Source: CAD feature listing. Evaluate the final solid. Frame: model axes, mm. A direction names the side the tool comes from. Round coordinates to 2 decimals unless told otherwise and drop trailing zeros. Loops run counter-clockwise (first coordinate to the right, second up) from the corner with the lowest first, then second, coordinate; pieces in that order, holes last. Notation, with made-up numbers: (84, 40) -> (89, 40) arc R12 ccw to (89, 61) -> close; hole circle Ø1 at (15.5, 87.5). An arc over 180 degrees is marked (long way). Write item = value, one per line.
from build123d import *

# Parameters (mm, degrees)
F0_W     = 41.6900217533
F0_H     = 40.332518518
F1_DEPTH = 560
F2_DEPTH = 600
F3_DEPTH = 2000
F4_T     = -18


with BuildPart() as f1:
    # F0 (on Front) → F1 (new body)
    with BuildSketch(Plane.XZ):
        with Locations((20.8450108767, 20.166259259)):
            Rectangle(F0_W, F0_H)
    extrude(amount=F1_DEPTH)

    # F2 (add): a face of the model
    f2_faces = [f1.faces().sort_by_distance(p)[0] for p in [
        (0, -280, 20.166259259),
    ]]
    extrude(f2_faces, amount=-F2_DEPTH)

    # F3 (add): a face of the model
    f3_faces = [f1.faces().sort_by_distance(p)[0] for p in [
        (300, -280, 0),
    ]]
    extrude(f3_faces, amount=-F3_DEPTH)

    # F4
    f4_openings = [f1.faces().sort_by_distance(p)[0] for p in [
        (300, -560, 1000),
    ]]
    offset(amount=F4_T, openings=f4_openings)


solid = f1.part
1. Section query A-A (z = 1758.5). Return the cut outline in (x, y), then the cut area to 3 significant figures.
Evaluation:
outline = (0, -560) -> (18, -560) -> (18, -18) -> (582, -18) -> (582, -560) -> (600, -560) -> (600, 0) -> (0, 0) -> close
area = 30,300 mm²
2. Section query B-B (y = -304.5). Return the cut outline in (x, z).
Evaluation:
outline = (0, 0) -> (600, 0) -> (600, 2000) -> (0, 2000) -> close; hole (18, 18) -> (582, 18) -> (582, 1982) -> (18, 1982) -> close
3. Mould query, pull axis X, two halves, no side actions, for faces 3 (the face through (296, -276, 2000)), 4 (the face through (296, -18, 1014)), 5 (the face through (600, -276, 986)). Classes: released by +X, released by -X, zero draft, split by the parting line, or undercut.
Evaluation:
face_3 = zero draft
face_4 = undercut
face_5 = released by +X
4. Line query: probe 1 along Z at (x, y) = (402.5, -345.5); probe 2 along X at (y, z) = (-26, 1506); probe 3 along Y at (x, z) = (417.5, 1446). Output: solid intervals per line, ascending. Write a range as from..to.
Evaluation:
probe_1 = 0..18, 1982..2000
probe_2 = 0..18, 582..600
probe_3 = -18..0
5. Set-up query: faces 1 (the face through (296, -285, 1982)), 2 (the face through (10, -560, 1005)). Return all of +Z, -Z, +X, -X, +Y, -Y with unobstructed straight access to the full face (end or side cutting, diameter ignored); none if empty.
Evaluation:
face_1 = -Y
face_2 = +Z, -Z, +X, -X, -Y
6. Section query C-C (x = 351). Return the cut outline in (y, z), then the cut area to 3 significant figures.
Evaluation:
outline = (-560, 0) -> (0, 0) -> (0, 2000) -> (-560, 2000) -> (-560, 1982) -> (-18, 1982) -> (-18, 18) -> (-560, 18) -> close
area = 55,500 mm²
